```python
from build123d import *

# Parameters (mm, degrees)
F1_DEPTH = 311.15
F2_R     = 5.08
F3_R     = 11.1125
F4_DEPTH = 25.4


with BuildPart() as f1:
    # F0 (on Front) → F1 (new body, symmetric)
    with BuildSketch(Plane.XZ):
        Polygon((-38.1, -38.1), (38.1, -38.1), (38.1, -31.75), (-31.75, -31.75), (-31.75, 38.1), (-38.1, 38.1), align=None)
    extrude(amount=F1_DEPTH, both=True)

    # F2
    f2_edges = [f1.edges().sort_by_distance(p)[0] for p in [
        (-31.75, 0, 38.1),
        (-31.75, 0, -31.75),
        (38.1, 0, -31.75),
    ]]
    fillet(f2_edges, radius=F2_R)

    # F3 (on face) → F4 (cut)
    with BuildSketch(Plane.YZ.offset(-31.75)):
        with Locations((260.35, 3.175)):
            Circle(F3_R)
        with Locations((-260.35, 3.175)):
            Circle(F3_R)
    extrude(amount=-F4_DEPTH, mode=Mode.SUBTRACT)


solid = f1.part
```
Could you check a few things on this model? Use its own coordinates, in mm. A direction names the side the tool comes from. Coordinates: 2 decimals unless noted, no trailing zeros. Loops run counter-clockwise (first coordinate to the right, second up) from the corner with the lowest first, then second, coordinate; pieces in that order, holes last.
1) Will these pins go through, and if not, where does the flat tip stop? pin 1 Ø6 at (y, z) = (147, -2.5) entering from +X; pin 2 Ø18 at (x, y) = (10, 78.5) entering from +Z; pin 3 Ø20 at (y, z) = (260.35, 3.175) entering from +X.
Reported:
pin 1: stops at x = -31.75
pin 2: stops at z = -31.75
pin 3: passes through
2) Imagine slicing it at C-C (z = -20.5). List the corners of the cut face in (x, y) for me.
Reported:
outline: (-38.1, -311.15) - (-31.75, -311.15) - (-31.75, 311.15) - (-38.1, 311.15) - close
3) Imagine slicing it at D-D (x = 4.5). List the corners of the cut face in (y, z) for me.
Reported:
outline: (-311.15, -38.1) - (311.15, -38.1) - (311.15, -31.75) - (-311.15, -31.75) - close
4) Thinking about a two-plate mould opening in Y: for faces 1 (the face through (-34, 311.15, -14)), 2 (the face through (-31.75, -4, 3)), 3 (the face through (-34.88, -249.75, 6.51)), 4 (the face through (-34.88, 270.95, 6.51)), which applies, released by +Y, released by -Y, zero draft, split by the parting line, or undercut?
Reported:
face 1: released by +Y
face 2: zero draft
face 3: undercut
face 4: undercut
5) Which directions (+Z, -Z, +X, -X, +Y, -Y) give clear straight access to the entire face, cutting with the end or side of a thin tool? Please do faces 5 (the face through (-34, -311.15, -14)), 6 (the face through (4, -4, -31.75)).
Reported:
face 5: +Z, -Z, +X, -X, -Y
face 6: +Z, +X, +Y, -Y
6) Imagine slicing it at B-B (y = -230.5). List the corners of the cut face in (x, z) for me, and give its area (3 significant figures).
Reported:
outline: (-38.1, -38.1) - (38.1, -38.1) - (38.1, -36.83) arc R5.08 ccw to (33.02, -31.75) - (-26.67, -31.75) arc R5.08 cw to (-31.75, -26.67) - (-31.75, 33.02) arc R5.08 ccw to (-36.83, 38.1) - (-38.1, 38.1) - close
area: 922 mm2
7) Imagine slicing it at A-A (y = 260.35). List the corners of the cut face in (x, z) for me.
Reported:
outline: (-38.1, -38.1) - (38.1, -38.1) - (38.1, -36.83) arc R5.08 ccw to (33.02, -31.75) - (-26.67, -31.75) arc R5.08 cw to (-31.75, -26.67) - (-31.75, -7.94) - (-38.1, -7.94) - close; (-38.1, 14.29) - (-31.75, 14.29) - (-31.75, 33.02) arc R5.08 ccw to (-36.83, 38.1) - (-38.1, 38.1) - close
8) Please list where these lines run through material, in increasing order: line 1 along Z through (x, y) = (-36.5, -260.35); line 2 along Z through (x, y) = (-36, -260.35); line 3 along Z through (x, y) = (-10, -204.5).
Reported:
line 1: z = -38.1 to -7.94, 14.29 to 38.09
line 2: z = -38.1 to -7.94, 14.29 to 38.03
line 3: z = -38.1 to -31.75
